from build123d import *

# Parameters (mm, degrees)
SCALE1_SCALE            = 10
CUT_EXTRUDE1_DEPTH      = 10
CUT_EXTRUDE1_DEPTH_BACK = 10
SKETCH4_R               = 5


with BuildPart() as part:
    # Sketch1 → Revolve1 (revolve)
    with BuildSketch(Plane.XY, mode=Mode.PRIVATE) as revolve1_sk:
        Polygon((-22.439160201, 47.327777778), (-22.439160201, 45.464860395), (-21.56053595, 45.464860395), (-21.56053595, 39.827777778), (-20.955555556, 39.827777778), (-20.955555556, 47.327777778), (-14.355555556, 47.327777778), (-14.355555556, 48.827777778), (-31.355555556, 48.827777778), (-31.355555556, 47.327777778), align=None)
    revolve(revolve1_sk.sketch.rotate(Axis((-14.355555556, 34.827777778, 0), (-1, 0, 0)), 90), axis=Axis((-14.355555556, 34.827777778, 0), (-1, 0, 0)))


with BuildPart() as part_1:
    # Scale1: scaled about (-22.654736369, 34.827777778, 0)
    add(part.part.scale(SCALE1_SCALE).moved(Location((203.892627321, -313.450000002, 0))))

    # Sketch4 → Cut-Extrude1 (cut, two sides: drawn at the far end of the back side and taken through both)
    with BuildSketch(Plane.ZY.offset(11.712732179).offset(-CUT_EXTRUDE1_DEPTH_BACK)):
        with Locations(Location((-70, 34.827777778, 0), (0, 0, 180))):
            Circle(SKETCH4_R)
        with Locations(Location((0, 104.827777778, 0), (0, 0, 180))):
            Circle(SKETCH4_R)
        with Locations(Location((70, 34.827777778, 0), (0, 0, 180))):
            Circle(SKETCH4_R)
        with Locations(Location((0, -35.172222222, 0), (0, 0, 180))):
            Circle(SKETCH4_R)
    extrude(amount=CUT_EXTRUDE1_DEPTH + CUT_EXTRUDE1_DEPTH_BACK, mode=Mode.SUBTRACT)


solid = part_1.part
Could you check a few things on this model? Use its own coordinates, in mm. A direction names the side the tool comes from. Coordinates: 2 decimals unless noted, no trailing zeros. Order: outer loops, then holes, each group sorted by start corner. A loop starts at its lowest first (then second) coordinate and runs counter-clockwise, first axis right, second up. Notation, with made-up numbers: (18, 89.5) - (34, 89.5) arc R29 ccw to (34, 124.5) - close; hole circle Ø11 at (73, 76). An arc over 180 degrees is marked (long way). Answer in a Markdown table with one row per item. Add a question column.
(1) On a 3-axis mill with a long thin cutter (end or side, diameter ignored), from which of +Z, -Z, +X, -X, +Y, -Y can I reach the whole of each face in a straight line? I mean faces 1 (the face through (27.799, 156.855, 27.098)), 2 (the face through (-20.499, -31, 84)), 3 (the face through (-8.645, 100.612, -2.688)). Say none if no direction works.
(2) If we mould it in two halves opening along Y, with no side actions, what happens to faces 4 (the face through (-109.663, -80, 53)), 5 (the face through (-11.713, 81, -22)), 6 (the face through (-25.85, 171.5, 30.35))? For each: released by +Y, released by -Y, zero draft, split by the parting line, or undercut.
(3) If we section it at B-B, the plane z = -43: Please give me the cut outline in (x, y).
(4) If we section it at D-D, the plane y = -85.5: Please give me the cut outline in (x, z), then the cut area to 3 significant figures.
(5) Will these pins go through, and if not, where does the flat tip stop? pin 1 (11.5 mm diameter, centred on y = 34.83, z = 70, fed in from -X); pin 2 (1.5 mm diameter, centred on x = 2.5, y = -24, fed in from +Z); pin 3 (8 mm diameter, centred on x = 5.5, y = 56.5, fed in from +Z); pin 4 (8 mm diameter, centred on y = -35.17, z = 0, fed in from -X).
(6) If we section it at A-A, the plane z = 0: Please give me the cut outline in (x, y), then the cut area to 3 significant figures.
(7) I need wall thicknesses on L1, parallel to Y at x = -9.5, z = 0; L2, parallel to Y at x = -18, z = 0; L3, parallel to X at y = 127.5, z = -31.5. Which ranges of each line are inside material? Lowest first, please.
(8) If we section it at C-C, the plane y = 44: Please give me the cut outline in (x, z).
Results are:
| question | item | result |
|---|---|---|
| 1 | face 1 | +X |
| 1 | face 2 | -X |
| 1 | face 3 | +X, -X |
| 2 | face 4 | zero draft |
| 2 | face 5 | undercut |
| 2 | face 6 | split by the parting line |
| 3 | outline | (-109.66, -98.41) - (60.34, -98.41) - (60.34, -82.54) - (-5.66, -82.54) - (-5.66, 9.31) - (-11.71, 9.31) - (-11.71, -62.46) - (-20.5, -62.46) - (-20.5, -82.54) - (-109.66, -82.54) - close; (-109.66, 152.2) - (-20.5, 152.2) - (-20.5, 132.12) - (-11.71, 132.12) - (-11.71, 60.34) - (-5.66, 60.34) - (-5.66, 152.2) - (60.34, 152.2) - (60.34, 168.06) - (-109.66, 168.06) - close |
| 4 | outline | (-109.66, -71.56) - (60.34, -71.56) - (60.34, -33.86) - (-5.66, -33.86) - (-5.66, 33.86) - (60.34, 33.86) - (60.34, 71.56) - (-109.66, 71.56) - (-109.66, 33.86) - (-20.5, 33.86) - (-20.5, -33.86) - (-109.66, -33.86) - close |
| 4 | area | 13,800 mm2 |
| 5 | pin 1 | stops at x = -11.71 |
| 5 | pin 2 | stops at z = 127.39 |
| 5 | pin 3 | stops at z = 138.88 |
| 5 | pin 4 | passes through |
| 6 | outline | (-109.66, -105.17) - (60.34, -105.17) - (60.34, -90.17) - (-5.66, -90.17) - (-5.66, -40.17) - (-11.71, -40.17) - (-11.71, -71.54) - (-20.5, -71.54) - (-20.5, -90.17) - (-109.66, -90.17) - close; (-109.66, 159.83) - (-20.5, 159.83) - (-20.5, 141.2) - (-11.71, 141.2) - (-11.71, 109.83) - (-5.66, 109.83) - (-5.66, 159.83) - (60.34, 159.83) - (60.34, 174.83) - (-109.66, 174.83) - close; (-11.71, -30.17) - (-5.66, -30.17) - (-5.66, -15.17) - (-11.71, -15.17) - close; (-11.71, 84.83) - (-5.66, 84.83) - (-5.66, 99.83) - (-11.71, 99.83) - close |
| 6 | area | 6,210 mm2 |
| 7 | L1 | y = -105.17 to -40.17, -30.17 to -15.17, 84.83 to 99.83, 109.83 to 174.83 |
| 7 | L2 | y = -105.17 to -71.54, 141.2 to 174.83 |
| 7 | L3 | x = -11.71 to -5.66 |
| 8 | outline | (-109.66, -139.7) - (60.34, -139.7) - (60.34, -124.66) - (-5.66, -124.66) - (-5.66, -49.15) - (-11.71, -49.15) - (-11.71, -105.97) - (-20.5, -105.97) - (-20.5, -124.66) - (-109.66, -124.66) - close; (-109.66, 124.66) - (-20.5, 124.66) - (-20.5, 105.97) - (-11.71, 105.97) - (-11.71, 49.15) - (-5.66, 49.15) - (-5.66, 124.66) - (60.34, 124.66) - (60.34, 139.7) - (-109.66, 139.7) - close |
